Check sheet for the modelled part. Datum: model origin and axes. Units: mm. Round coordinates to 2 decimals unless told otherwise and drop trailing zeros. Loops run counter-clockwise (first coordinate to the right, second up) from the corner with the lowest first, then second, coordinate; pieces in that order, holes last. Notation, with made-up numbers: (-3, 40.5) - (9, 40.5) arc R21 ccw to (9, 57.5) - close; hole circle Ø2 at (-0.75, -30.5). An arc over 180 degrees is marked (long way). Put each result on its own line as item: value.
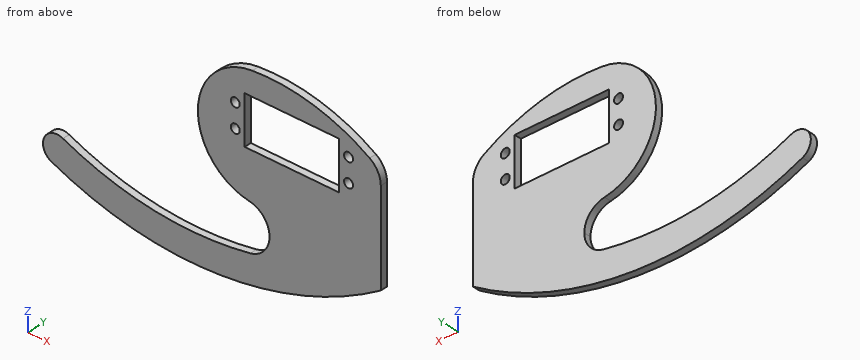
Autodesk Inventor part; units mm, degrees
ref_plane "YZ Plane" through (0, 0, 0) normal (1, 0, 0) x (0, 1, 0)
ref_plane "XZ Plane" through (0, 0, 0) normal (0, 1, 0) x (-1, 0, 0)
ref_plane "XY Plane" through (0, 0, 0) normal (0, 0, 1) x (1, 0, 0)
sketch "Sketch1" plane through (0, 0, 0) normal (0, 1, 0) x (-1, 0, 0)
  arc A0 (-1.4142, 9.8995) -> (-10, 0) centre (0, 0) ccw
  line L0 (-39.5, 50.25) -> (0.5, 50.25)
  line L1 (0.5, 50.25) -> (0.5, 29.75)
  line L2 (0.5, 29.75) -> (-39.5, 29.75)
  line L3 (-39.5, 29.75) -> (-39.5, 50.25)
  line L4 (-39.5, 50.25) -> (0.5, 29.75) construction
  line L5 (0.5, 50.25) -> (-39.5, 29.75) construction
  line L6 (-10, 40) -> (-19.5, 40) construction
  circle A1 centre (4.5, 35) radius 1.9
  circle A2 centre (4.5, 45) radius 1.9
  line L7 (4.5, 45) -> (4.5, 35) construction
  circle A3 centre (-43.5, 45) radius 1.9
  circle A4 centre (-43.5, 35) radius 1.9
  line L8 (-43.5, 45) -> (-43.5, 35) construction
  line L9 (-43.5, 40) -> (-19.5, 40) construction
  line L10 (-10, 40) -> (4.5, 40) construction
  line L11 (-43.5, 45) -> (4.5, 45) construction
  line L12 (-43.5, 35) -> (4.5, 35) construction
  line L13 (-19.5, 40) -> (-19.5, 45) construction
  circle A5 centre (-10, 40) radius 9.75 construction
  circle A6 centre (-29, 40) radius 9.75 construction
  arc A7 (-2.7044, 60.2512) -> (-52.4397, 48.5007) centre (-10, -20) ccw
  arc A8 (-1.4142, 9.8995) -> (-2.7044, 60.2512) centre (-5, 35) ccw
  line L14 (-57.1731, 40) -> (-57.1731, 0)
  line L15 (-57.1731, 0) -> (0, 0) construction
  arc A9 (-52.4397, 48.5007) -> (-57.1731, 40) centre (-47.1731, 40) ccw
  line L16 (0, 0) -> (10, 0) construction
  line L17 (-10, 0) -> (-57.1731, 0) construction
  arc A10 (-10, 0) -> (-1.4142, -9.8995) centre (0, 0) ccw
  arc A11 (-1.8715, -9.8233) -> (77.546, -0.5248) centre (23.0596, 121.0399) ccw
  arc A12 (82.454, -11.4752) -> (77.546, -0.5248) centre (80, -6) ccw
  arc A13 (-57.1731, 0) -> (82.454, -11.4752) centre (23.0596, 121.0399) ccw
  line L18 (0, 0) -> (100, 0) construction
  point P0 (-57.1731, 45.3313)
  point P1 (-5, -35)
  dimension "d0" = 20
  dimension "d1" = 40
  dimension "d2" = 20.5
  dimension "d4" = 48
  dimension "d5" = 3.8
  dimension "d6" = 10
  dimension "d7" = 19.5
  dimension "d8" = 10
  dimension "d9" = 40
  dimension "d11" = 10.5
  dimension "d12" = 35
  dimension "d13" = 5
  dimension "d16" = 10
  dimension "d17" = 20
  dimension "d18" = 10
  dimension "d19" = 40
  dimension "d47" = 12
  dimension "d48" = 100
  dimension "d49" = 80
  dimension "d60" = 14.5
extrude "Extrusion1" add sketch "Sketch1" along normal blind 3
equation "\"d11\" = d3"
properties part number "wstepna_geometria_wersja_2"
Item 1: Go/stop test with flat-tipped pins: pin 1 (1.5 mm diameter, centred on x = -25, y = 2, fed in from +Z); pin 2 (1.5 mm diameter, centred on x = 22, y = 1, fed in from +Z). Record where each tip stops, or that it passes through.
Filled sheet:
pin 1: z = -12.15
pin 2: z = 59.79
Item 2: Section check A-A on y = 0.45. Enter the section's corners in (x, z), then the cut area to 3 significant figures.
Filled sheet:
outline: (-82.45, -11.48) arc R145.22 ccw to (57.17, 0) - (57.17, 40) arc R10 ccw to (52.44, 48.5) arc R80.58 ccw to (2.7, 60.25) arc R25.36 ccw to (1.41, 9.9) arc R10 cw to (10, 0) arc R10 cw to (1.87, -9.82) arc R133.22 cw to (-77.55, -0.52) arc R6 ccw to start; hole circle Ø3.8 at (-4.5, 35); hole circle Ø3.8 at (-4.5, 45); hole (-0.5, 29.75) - (39.5, 29.75) - (39.5, 50.25) - (-0.5, 50.25) - close; hole circle Ø3.8 at (43.5, 35); hole circle Ø3.8 at (43.5, 45)
area: 4,770 mm²
Item 3: Thickness scan on line 1 (Z direction, x = -4.5, y = 1.4); line 2 (Z direction, x = 8.5, y = 2); line 3 (Z direction, x = 3.5, y = 2.65). Record the ranges inside material, lowest first. Write a range as from..to.
Filled sheet:
line 1: -22.99..-10.88, 11.49..33.1, 36.9..43.1, 46.9..58.51
line 2: -20.71..-5.27, 5.27..29.75, 50.25..60.57
line 3: -21.73..-9.37, 9.37..29.75, 50.25..60.32
Item 4: Section check C-C on z = 45. Enter the section's corners in (x, y), then the cut area to 3 significant figures.
Filled sheet:
outline: (-18.3, 0) - (-6.4, 0) - (-6.4, 3) - (-18.3, 3) - close; (-2.6, 0) - (-0.5, 0) - (-0.5, 3) - (-2.6, 3) - close; (39.5, 0) - (41.6, 0) - (41.6, 3) - (39.5, 3) - close; (45.4, 0) - (55.83, 0) - (55.83, 3) - (45.4, 3) - close
area: 79.6 mm²
Item 5: Section check B-B on x = -16. Enter the section's corners in (y, z), then the cut area to 3 significant figures.
Filled sheet:
outline: (0, -24.01) - (3, -24.01) - (3, -11.99) - (0, -11.99) - close; (0, 20.79) - (3, 20.79) - (3, 49.21) - (0, 49.21) - close
area: 121 mm²
Item 6: Section check D-D on x = 24.5. Enter the section's corners in (y, z).
Filled sheet:
outline: (0, -16.17) - (3, -16.17) - (3, 29.75) - (0, 29.75) - close; (0, 50.25) - (3, 50.25) - (3, 59.27) - (0, 59.27) - close
